from build123d import *

# Parameters (mm, degrees)
SKETCH1_W             = 49.2125
SKETCH1_H             = 49.2125
BOSS_EXTRUDE1_DEPTH   = 736.6
BOSS_EXTRUDE1_2_DEPTH = 736.6
SKETCH2_W             = 49.2125
SKETCH2_H             = 49.2125
BOSS_EXTRUDE2_DEPTH   = 458.7875
FILLET1_R             = 1.016


with BuildPart() as part:
    # Sketch1 → Boss-Extrude1 (new body)
    with BuildSketch(Plane(origin=(0, 0, 0), x_dir=(1, 0, 0), z_dir=(0, 1, 0))):
        with Locations((-432.59375, 229.39375)):
            Rectangle(SKETCH1_W, SKETCH1_H)
    extrude(amount=BOSS_EXTRUDE1_DEPTH)



with BuildPart() as body_2:
    # Sketch1 → Boss-Extrude1 2 (new body)
    with BuildSketch(Plane(origin=(0, 0, 0), x_dir=(1, 0, 0), z_dir=(0, 1, 0))):
        with Locations((-432.59375, -229.39375)):
            Rectangle(SKETCH1_W, SKETCH1_H)
    extrude(amount=BOSS_EXTRUDE1_2_DEPTH)


with BuildPart() as part_1:
    add(part.part)

    add(body_2.part)  # Boss-Extrude2 merges body 2
    # Sketch2 → Boss-Extrude2 (add)
    with BuildSketch(Plane.XY.offset(-204.7875)):
        with Locations((-432.59375, 24.60625)):
            Rectangle(SKETCH2_W, SKETCH2_H)
    extrude(amount=BOSS_EXTRUDE2_DEPTH)

    # Fillet1
    fillet1_edges = [part_1.edges().sort_by_distance(p)[0] for p in [
        (-407.9875, 736.6, -229.39375),
        (-432.59375, 49.2125, 204.7875),
        (-407.9875, 49.2125, 0),
        (-432.59375, 49.2125, -204.7875),
        (-457.2, 49.2125, 0),
        (-432.59375, 736.6, -254),
        (-407.9875, 392.90625, 204.7875),
        (-432.59375, 0, 254),
        (-457.2, 368.3, 254),
        (-407.9875, 368.3, 254),
        (-457.2, 392.90625, 204.7875),
        (-432.59375, 736.6, 254),
        (-407.9875, 736.6, 229.39375),
        (-432.59375, 736.6, 204.7875),
        (-457.2, 736.6, 229.39375),
        (-457.2, 736.6, -229.39375),
        (-432.59375, 0, -254),
        (-407.9875, 0, 0),
        (-457.2, 0, 0),
        (-457.2, 368.3, -254),
        (-407.9875, 368.3, -254),
        (-407.9875, 392.90625, -204.7875),
        (-457.2, 392.90625, -204.7875),
        (-432.59375, 736.6, -204.7875),
    ]]
    fillet(fillet1_edges, radius=FILLET1_R)


solid = part_1.part
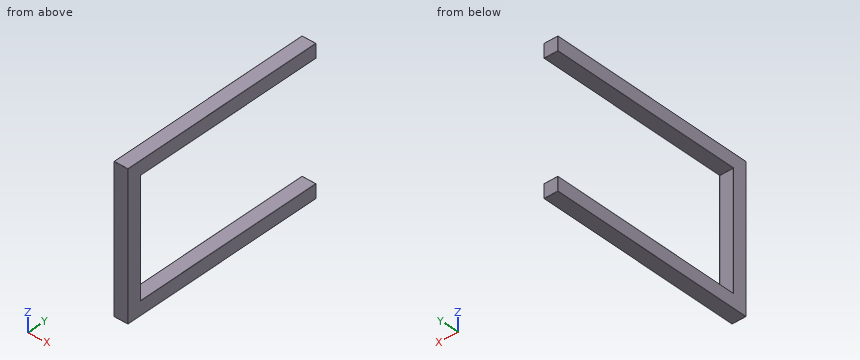
Could you check a few things on this model? Use its own coordinates, in mm. Give positions to 0.01 mm unless a question says otherwise; leave off trailing zeros. Write each loop counter-clockwise with the first axis right and the second up, starting at its lowest first coordinate (ties: lowest second). Pieces come first, ordered by that corner, then holes. Notation, with made-up numbers: (42, 37) -> (95, 37) arc R23 ccw to (95, 52) -> close; hole circle Ø3 at (66, 38). An arc over 180 degrees is marked (long way). Answer as CSV lines item,"result". Start each with the question number.
(1) If we section it at A-A, the plane y = 176: Write out the boundary of the cut face in (x, z).
(2) If we section it at B-B, the plane x = -422: Write out the boundary of the cut face in (y, z).
(3) Please list where these lines run through material, in increasing order: line 1 (Z direction, x = -420, y = 303); line 2 (Y direction, x = -438.5, z = 89).
(4) If we section it at C-C, the plane z = 178.5: Write out the boundary of the cut face in (x, y), and give its area (3 significant figures).
(5) I'm going to push a flat-ended pin straight in: pin 1 Ø1.5 at (x, z) = (-449, 145.5) entering from +Y. Where does the tip first touch, or does it pass through?
Answer list:
1,outline,"(-457.2, -252.98) arc R1.02 ccw to (-456.18, -254) -> (-409, -254) arc R1.02 ccw to (-407.99, -252.98) -> (-407.99, -205.8) arc R1.02 ccw to (-409, -204.79) -> (-456.18, -204.79) arc R1.02 ccw to (-457.2, -205.8) -> close; (-457.2, 205.8) arc R1.02 ccw to (-456.18, 204.79) -> (-409, 204.79) arc R1.02 ccw to (-407.99, 205.8) -> (-407.99, 252.98) arc R1.02 ccw to (-409, 254) -> (-456.18, 254) arc R1.02 ccw to (-457.2, 252.98) -> close"
2,outline,"(0, -252.98) arc R1.02 ccw to (1.02, -254) -> (735.58, -254) arc R1.02 ccw to (736.6, -252.98) -> (736.6, -205.8) arc R1.02 ccw to (735.58, -204.79) -> (50.23, -204.79) arc R1.02 cw to (49.21, -203.77) -> (49.21, 203.77) arc R1.02 cw to (50.23, 204.79) -> (735.58, 204.79) arc R1.02 ccw to (736.6, 205.8) -> (736.6, 252.98) arc R1.02 ccw to (735.58, 254) -> (1.02, 254) arc R1.02 ccw to (0, 252.98) -> close"
3,line 1,"-254 to -204.79, 204.79 to 254"
3,line 2,"0 to 49.21"
4,outline,"(-457.2, 1.02) arc R1.02 ccw to (-456.18, 0) -> (-409, 0) arc R1.02 ccw to (-407.99, 1.02) -> (-407.99, 48.2) arc R1.02 ccw to (-409, 49.21) -> (-456.18, 49.21) arc R1.02 ccw to (-457.2, 48.2) -> close"
4,area,"2,420 mm^2"
5,pin 1,"y = 49.21"
